```python
from build123d import *

# Parameters (mm, degrees)
SUPERFICIE_EXTRUIR1_1_BACK  = 10
SUPERFICIE_EXTRUIR1_1_DEPTH = 20
DAR_ESPESOR1_T1             = 2
CROQUIS2_R                  = 2
CORTAR_EXTRUIR1_DEPTH       = 2
REDONDEO1_R                 = 10
CROQUIS3_R                  = 2
CORTAR_EXTRUIR2_DEPTH       = 2


with BuildPart() as body_1:
    # Superficie-Extruir1: a surface, the sketch's curves swept straight by 20 mm
    with BuildLine(Plane.XY.offset(-SUPERFICIE_EXTRUIR1_1_BACK), mode=Mode.PRIVATE) as superficie_extruir1_1_path:
        Line((-51, 0), (-51, 35))
        Line((-51, 35), (51, 35))
        Line((51, 35), (51, 0))
        Line((51, 0), (51, -16))
    superficie_extruir1_1 = Shell.extrude(superficie_extruir1_1_path.wire(), (0 * SUPERFICIE_EXTRUIR1_1_DEPTH, 0 * SUPERFICIE_EXTRUIR1_1_DEPTH, 1 * SUPERFICIE_EXTRUIR1_1_DEPTH))
    add(Solid.thicken(superficie_extruir1_1, DAR_ESPESOR1_T1))

    # Croquis2 → Cortar-Extruir1 (cut)
    with BuildSketch(Plane.ZY.offset(53)):
        with Locations((0, 10.5)):
            Circle(CROQUIS2_R)
        with BuildLine():
            Line((-10, 10.5), (-10, 0))
            Line((-10, 0), (10, 0))
            Line((10, 0), (10, 10.5))
            ThreePointArc((10, 10.5), (0, 0.5), (-10, 10.5))
        make_face()
    extrude(amount=-CORTAR_EXTRUIR1_DEPTH, mode=Mode.SUBTRACT)

    # Redondeo1
    redondeo1_edges = [body_1.edges().sort_by_distance(p)[0] for p in [
        (-51, 35, 0),
        (51, 35, 0),
        (53, 37, 0),
        (-53, 37, 0),
    ]]
    fillet(redondeo1_edges, radius=REDONDEO1_R)

    # Croquis3 → Cortar-Extruir2 (cut)
    with BuildSketch(Plane(origin=(53, 0, 0), x_dir=(0, 0, -1), z_dir=(1, 0, 0))):
        with Locations((0, -5.5)):
            Circle(CROQUIS3_R)
        with BuildLine():
            Line((-10, -5.5), (-10, -16))
            Line((-10, -16), (10, -16))
            Line((10, -16), (10, -5.5))
            ThreePointArc((10, -5.5), (0, -15.5), (-10, -5.5))
        make_face()
    extrude(amount=-CORTAR_EXTRUIR2_DEPTH, mode=Mode.SUBTRACT)


solid = body_1.part
```
Source: CAD feature listing. Evaluate the final solid. Frame: model axes, mm. A direction names the side the tool comes from. Coordinates: 2 decimals unless noted, no trailing zeros. Loops run counter-clockwise (first coordinate to the right, second up) from the corner with the lowest first, then second, coordinate; pieces in that order, holes last. Notation, with made-up numbers: M 7.5,-34 L 62.5,-34 A19 ccw 62.5,-24 Z; hole C 80.5,25.5 d2. An arc over 180 degrees is marked long. Use a Markdown table: item, result. Add a question column.
Q1. Draft query along X for faces 6 (the flat face through (-1, 35, 0)), 7 (the flat face through (53, 6, 0)), 8 (the cylindrical face through (-50.15, 33.99, -0.14)), 9 (the cylindrical face through (52, -15.5, -0.2)). Return one class per face: pulls with the +X half, pulls with the -X half, needs draft (parallel to the pull), parting line crosses it, or undercut.
Q2. Section query A-A, the plane z = 0. Return loops of the section in (x, y).
Q3. Section query B-B, the plane x = 34.5. Return loops of the section in (y, z), and give its area (3 significant figures).
Q4. Material intervals for L1, parallel to X at y = 20, z = -9; L2, parallel to Y at x = 22.5, z = -7; L3, parallel to X at y = 0, z = 4.75, sorted ascending.
Q5. First-contact query: pin 1 (3 mm diameter, centred on x = 1.5, z = -4, fed in from -Y); pin 2 (3.5 mm diameter, centred on y = -5.5, z = 0, fed in from +X). Flat tips, straight axial feed; report the tip coordinate or a pass-through.
Q6. Access query for faces 1 (the flat face through (-12, 36, -10)), 2 (the cylindrical face through (-52.014, 12.483, -0.26)), 3 (the flat face through (51, 5, 0)), 4 (the cylindrical face through (-52, 0.5, 0.2)), 5 (the flat face through (-1, 37, 0)). Directions: +Z, -Z, +X, -X, +Y, -Y. A direction counts if a zero-diameter tool reaches every point of the face in a straight line with its end or side. Return the directions, or none.
Q7. Section query C-C, the plane z = 7.5. Return loops of the section in (x, y), and give its area (3 significant figures).
Result:
| question | item | result |
|---|---|---|
| 1 | face 6 | undercut |
| 1 | face 7 | pulls with the +X half |
| 1 | face 8 | pulls with the -X half |
| 1 | face 9 | needs draft |
| 2 | outline | M -53,0.5 L -51,0.5 L -51,8.5 L -53,8.5 Z; M -53,12.5 L -51,12.5 L -51,25 A10 cw -41,35 L 41,35 A10 cw 51,25 L 51,-3.5 L 53,-3.5 L 53,27 A10 ccw 43,37 L -43,37 A10 ccw -53,27 Z; M 51,-15.5 L 53,-15.5 L 53,-7.5 L 51,-7.5 Z |
| 3 | outline | M 35,-10 L 37,-10 L 37,10 L 35,10 Z |
| 3 | area | 40.0 mm2 |
| 4 | L1 | x = -53 to -51, 51 to 53 |
| 4 | L2 | y = 35 to 37 |
| 4 | L3 | x = 51 to 53 |
| 5 | pin 1 | stops at y = 35 |
| 5 | pin 2 | passes through |
| 6 | face 1 | -Z, +X, -X, +Y, -Y |
| 6 | face 2 | -X |
| 6 | face 3 | +Z, -Z, -Y |
| 6 | face 4 | -X, -Y |
| 6 | face 5 | +Z, -Z, +X, -X, +Y |
| 7 | outline | M -53,3.89 L -51,3.89 L -51,25 A10 cw -41,35 L 41,35 A10 cw 51,25 L 51,-12.11 L 53,-12.11 L 53,27 A10 ccw 43,37 L -43,37 A10 ccw -53,27 Z |
| 7 | area | 368 mm2 |
